from build123d import *

# Parameters (mm, degrees)
SKETCH1_W           = 355.6
SKETCH1_H           = 114.3
BOSS_EXTRUDE1_DEPTH = 3
SKETCH3_R           = 3.175
CUT_EXTRUDE1_DEPTH  = 3
CUT_EXTRUDE2_REACH  = 188.783
SKETCH4_W           = 355.6
SKETCH4_H           = 25.4


with BuildPart() as part:
    # Sketch1 → Boss-Extrude1 (new body)
    with BuildSketch(Plane.XY):
        Rectangle(SKETCH1_W, SKETCH1_H)
    extrude(amount=BOSS_EXTRUDE1_DEPTH)

    # Sketch3 → Cut-Extrude1 (cut)
    with BuildSketch(Plane.XY.offset(3)):
        with Locations((-60.325, 0)):
            Circle(SKETCH3_R)
        Circle(SKETCH3_R)
        with Locations((-150.749, 20)):
            Circle(SKETCH3_R)
    cut_extrude1 = extrude(amount=-CUT_EXTRUDE1_DEPTH, mode=Mode.SUBTRACT)

    # Mirror3: Cut-Extrude1 across plane
    add(cut_extrude1.mirror(Plane(origin=(0, 0, 0), x_dir=(0, 0, 1), z_dir=(1, 0, 0))), mode=Mode.SUBTRACT)

    # Sketch4 → Cut-Extrude2 (cut, up to next)
    with BuildSketch(Plane(origin=(0, 0, 0), x_dir=(-1, 0, 0), z_dir=(0, 0, -1)), mode=Mode.PRIVATE) as cut_extrude2_sk1:
        with Locations((0, -44.45)):
            Rectangle(SKETCH4_W, SKETCH4_H)
    cut_extrude2_tool1 = extrude(cut_extrude2_sk1.sketch, amount=-CUT_EXTRUDE2_REACH, mode=Mode.PRIVATE) & part.part
    add(cut_extrude2_tool1.solids().sort_by_distance((0, -44.45, 0))[0], mode=Mode.SUBTRACT)


solid = part.part
Source: CAD feature listing. Evaluate the final solid. Frame: model axes, mm. Round coordinates to 2 decimals unless told otherwise and drop trailing zeros. Order: outer loops, then holes, each group sorted by start corner. A loop starts at its lowest first (then second) coordinate and runs counter-clockwise, first axis right, second up. Notation, with made-up numbers: (41.5, -29) - (69.5, -29) arc R15 ccw to (69.5, -21) - close; hole circle Ø11 at (-10, -12.75). An arc over 180 degrees is marked (long way). Use a Markdown table: item, result. Add a question column.
1. Mould query, pull axis X, two halves, no side actions, for faces 1 (the flat face through (-2, 13, 3)), 2 (the cylindrical face through (153.92, 20.14, 1.52)). Classes: +X half, -X half, draft (parallel to the pull), parting line (faces both ways), or undercut.
2. Section query A-A (y = 0). Return the cut outline in (x, z) (3 decimals), then the cut area to 3 significant figures.
3. Line query: probe 1 along Y at (x, z) = (0, 1.7) (3 decimals); probe 2 along Y at (x, z) = (153, 2.65). Output: solid intervals per line, ascending.
4. Section query C-C (x = 0). Return the cut outline in (y, z) (3 decimals).
5. Section query B-B (y = 20). Return the cut outline in (x, z), then the cut area to 3 significant figures.
Derived:
| question | item | result |
|---|---|---|
| 1 | face 1 | draft |
| 1 | face 2 | undercut |
| 2 | outline | (-177.8, 0) - (-63.5, 0) - (-63.5, 3) - (-177.8, 3) - close; (-57.15, 0) - (-3.175, 0) - (-3.175, 3) - (-57.15, 3) - close; (3.175, 0) - (57.15, 0) - (57.15, 3) - (3.175, 3) - close; (63.5, 0) - (177.8, 0) - (177.8, 3) - (63.5, 3) - close |
| 2 | area | 1,010 mm2 |
| 3 | probe 1 | -31.75 to -3.175, 3.175 to 57.15 |
| 3 | probe 2 | -31.75 to 17.76, 22.24 to 57.15 |
| 4 | outline | (-31.75, 0) - (-3.175, 0) - (-3.175, 3) - (-31.75, 3) - close; (3.175, 0) - (57.15, 0) - (57.15, 3) - (3.175, 3) - close |
| 5 | outline | (-177.8, 0) - (-153.92, 0) - (-153.92, 3) - (-177.8, 3) - close; (-147.57, 0) - (147.57, 0) - (147.57, 3) - (-147.57, 3) - close; (153.92, 0) - (177.8, 0) - (177.8, 3) - (153.92, 3) - close |
| 5 | area | 1,030 mm2 |
